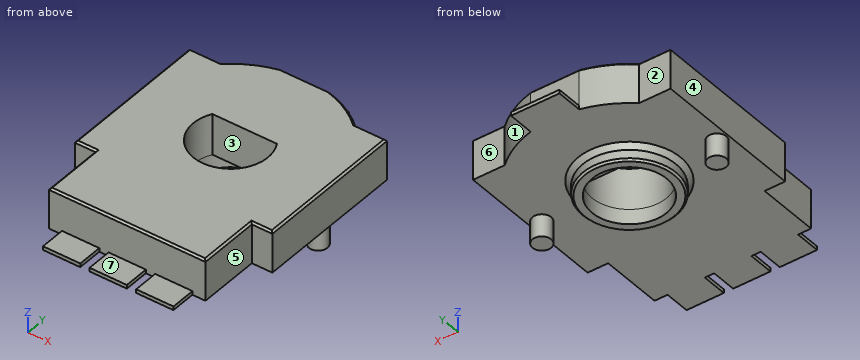
```python
from build123d import *

# Parameters (mm, degrees)
MODEL_R        = 0.5
MODEL_R_2      = 2.5
MODEL_R_3      = 2
EXTRUDE1_DEPTH = 2.2
SKETCH_W       = 1
SKETCH_H       = 1.35
EXTRUDE2_DEPTH = 0.2
SKETCH_2_R     = 2.5
SKETCH_2_R_2   = 2
EXTRUDE3_DEPTH = 0.8
SKETCH_3_R     = 0.5
EXTRUDE4_DEPTH = 1.2
CHAMFER1_SIZE  = 0.1
CHAMFER2_SIZE  = 0.25
CHAMFER3_SIZE  = 0.1
EXTRUDE5_START = -2.2
EXTRUDE5_DEPTH = 2.2


# Read off the part's stored shape, not the designer's step: Extrude5
with BuildPart() as part:
    # Model → Extrude1 (new body)
    # profile 1 of 5: a face of its own
    with BuildSketch(Plane.XY):
        with BuildLine():
            Line((0, 5.3), (-1.3, 5.3))
            ThreePointArc((-1.3, 5.3), (-2.523074038, 4.838811569), (-3.601388621, 4.1))
            Line((-3.601388621, 4.1), (-5.3, 4.1))
            Line((-5.3, 4.1), (-5.3, 0))
            Line((-5.3, 0), (-5.3, -4.05))
            Line((-5.3, -4.05), (-4.2, -4.05))
            Line((-4.2, -4.05), (-4.2, -7.35))
            Line((-4.2, -7.35), (0, -7.35))
            Line((0, -7.35), (4.2, -7.35))
            Line((4.2, -7.35), (4.2, -4.05))
            Line((4.2, -4.05), (5.3, -4.05))
            Line((5.3, -4.05), (5.3, 0))
            Line((5.3, 0), (5.3, 4.1))
            Line((5.3, 4.1), (3.601388621, 4.1))
            ThreePointArc((3.601388621, 4.1), (2.523074038, 4.838811569), (1.3, 5.3))
            Line((1.3, 5.3), (0, 5.3))
        make_face()
        with Locations((4.7, 0)):
            Circle(MODEL_R, mode=Mode.SUBTRACT)
        with Locations((-4.7, 0)):
            Circle(MODEL_R, mode=Mode.SUBTRACT)
        Circle(MODEL_R_2, mode=Mode.SUBTRACT)
    # profile 2 of 5: a face of its own
    with BuildSketch(Plane.XY):
        with Locations((-4.7, 0)):
            Circle(MODEL_R)
    # profile 3 of 5: a face of its own
    with BuildSketch(Plane.XY):
        with Locations((4.7, 0)):
            Circle(MODEL_R)
    # profile 4 of 5: a face of its own
    with BuildSketch(Plane.XY):
        Circle(MODEL_R_2)
        Circle(MODEL_R_3, mode=Mode.SUBTRACT)
    # profile 5 of 5: a face of its own
    with BuildSketch(Plane.XY):
        Circle(MODEL_R_3)
    extrude(amount=EXTRUDE1_DEPTH)

    # Sketch → Extrude2 (add)
    with BuildSketch(Plane.XY):
        Polygon((0, 6.7), (-1.3, 6.7), (-1.3, 5.3), (0, 5.3), (1.3, 5.3), (1.3, 6.7), align=None)
        with Locations((-2, -8.025)):
            Rectangle(SKETCH_W, SKETCH_H)
        with Locations((-3, -8.025)):
            Rectangle(SKETCH_W, SKETCH_H)
        Polygon((1, -8.7), (1, -7.35), (0, -7.35), (-1, -7.35), (-1, -8.7), (0, -8.7), align=None)
        with Locations((2, -8.025)):
            Rectangle(SKETCH_W, SKETCH_H)
        with Locations((3, -8.025)):
            Rectangle(SKETCH_W, SKETCH_H)
    extrude(amount=EXTRUDE2_DEPTH)

    # Sketch 2 → Extrude3 (add)
    with BuildSketch(Plane.XY):
        Circle(SKETCH_2_R)
        Circle(SKETCH_2_R_2, mode=Mode.SUBTRACT)
    extrude(amount=-EXTRUDE3_DEPTH)

    # Sketch 3 → Extrude4 (add)
    with BuildSketch(Plane.XY):
        with Locations((4.7, 0)):
            Circle(SKETCH_3_R)
        with Locations((-4.7, 0)):
            Circle(SKETCH_3_R)
    extrude(amount=-EXTRUDE4_DEPTH)

    # Chamfer1
    chamfer1_edges = [part.edges().sort_by_distance(p)[0] for p in [
        (-4.450694311, 4.1, 2.2),
        (-5.3, 0.025, 2.2),
        (-4.75, -4.05, 2.2),
        (-4.2, -5.7, 2.2),
        (0, -7.35, 2.2),
        (4.2, -5.7, 2.2),
        (0, 5.3, 2.2),
        (4.75, -4.05, 2.2),
        (5.3, 0.025, 2.2),
        (4.450694311, 4.1, 2.2),
        (2.523074038, 4.838811569, 2.2),
        (-2.523074038, 4.838811569, 2.2),
    ]]
    chamfer(chamfer1_edges, length=CHAMFER1_SIZE)

    # Chamfer2
    chamfer2_edges = [part.edges().sort_by_distance(p)[0] for p in [
        (-2.5, 0, 0),
    ]]
    chamfer(chamfer2_edges, length=CHAMFER2_SIZE)

    # Chamfer3
    chamfer3_edges = [part.edges().sort_by_distance(p)[0] for p in [
        (-2.5, 0, -0.8),
    ]]
    chamfer(chamfer3_edges, length=CHAMFER3_SIZE)

    # Extrude5 outline → Extrude5 (cut)
    with BuildSketch(Plane.XY.offset(2.2).offset(EXTRUDE5_START)):
        with BuildLine():
            ThreePointArc((-1.732050808, 1), (0, -2), (1.732050808, 1))
            Line((1.732050808, 1), (-1.732050808, 1))
        make_face()
    extrude(amount=EXTRUDE5_DEPTH, mode=Mode.SUBTRACT)


solid = part.part
```
CAD build for the part. Positions are in the model's coordinates, mm. Face numbers are marked on the shaded views. A direction names the side the tool comes from. Coordinates: 2 decimals unless noted, no trailing zeros. Write each loop counter-clockwise with the first axis right and the second up, starting at its lowest first coordinate (ties: lowest second). Pieces come first, ordered by that corner, then holes. Notation, with made-up numbers: (-4.5, -19) -> (35.5, -19) arc R22 ccw to (35.5, 8) -> close; hole circle Ø5 at (11.5, 45). An arc over 180 degrees is marked (long way). Return JSON: item names as keys, results as strings. Group by question number.
Q1. Cut at A-A, the plane z = 0.55. Give the cut face in (x, y), then the cut area to 3 significant figures.
Q2. Cut at B-B, the plane x = 0. Give the cut face in (y, z), then the cut area to 3 significant figures.
Q3. Cut at C-C, the plane y = -5. Give the cut face in (x, z), then the cut area to 3 significant figures.
Q4. Cut at D-D, the plane x = 4.7. Give the cut face in (y, z), then the cut area to 3 significant figures.
Q5. Drill centre lines: line 1 (Y direction, x = 1, z = -0.15); line 2 (X direction, y = 0, z = 1.2); line 3 (Z direction, x = -2.25, y = -4.5). Where is each one in solid material? Low to high.
Q6. Which spindle directions (+Z, -Z, +X, -X, +Y, -Y) get a long thin tool onto all of the face, cutting with end or side? Do the marked faces 5, 6 and 7. Say none if no direction does.
Q7. Pull direction X, two halves, no side cores. Call the marked faces 1, 2, 3 and 4: released by +X, released by -X, zero draft, split by the parting line, or undercut.
Q8. Flat gauge pins, fed straight in: pin 1 (1.5 mm diameter, centred on x = 0.5, y = 5.5, fed in from +Z); pin 2 (0.6 mm diameter, centred on x = -2, z = 1, fed in from -Y); pin 3 (2.5 mm diameter, centred on x = 0, y = 0, fed in from -Z); pin 4 (0.7 mm diameter, centred on x = 0, y = -8, fed in from +Z). Where does each tip first touch, or does it go through?
Returned:
{
 "1": {"outline": "(-5.3, -4.05) -> (-4.2, -4.05) -> (-4.2, -7.35) -> (4.2, -7.35) -> (4.2, -4.05) -> (5.3, -4.05) -> (5.3, 4.1) -> (3.6, 4.1) arc R5.46 ccw to (1.3, 5.3) -> (-1.3, 5.3) arc R5.46 ccw to (-3.6, 4.1) -> (-5.3, 4.1) -> close; hole (-1.73, 1) arc R2 ccw (long way) to (1.73, 1) -> close", "area": "110 mm2"},
 "2": {"outline": "(-8.7, 0) -> (-2.75, 0) -> (-2.5, -0.25) -> (-2.5, -0.7) -> (-2.4, -0.8) -> (-2, -0.8) -> (-2, 2.2) -> (-7.25, 2.2) -> (-7.35, 2.1) -> (-7.35, 0.2) -> (-8.7, 0.2) -> close; (1, 0) -> (2, 0) -> (2, -0.8) -> (2.4, -0.8) -> (2.5, -0.7) -> (2.5, -0.25) -> (2.75, 0) -> (6.7, 0) -> (6.7, 0.2) -> (5.3, 0.2) -> (5.3, 2.1) -> (5.2, 2.2) -> (1, 2.2) -> close", "area": "22.6 mm2"},
 "3": {"outline": "(-4.2, 0) -> (4.2, 0) -> (4.2, 2.1) -> (4.1, 2.2) -> (-4.1, 2.2) -> (-4.2, 2.1) -> close", "area": "18.5 mm2"},
 "4": {"outline": "(-4.05, 0) -> (-0.5, 0) -> (-0.5, -1.2) -> (0.5, -1.2) -> (0.5, 0) -> (4.1, 0) -> (4.1, 2.1) -> (4, 2.2) -> (-3.95, 2.2) -> (-4.05, 2.1) -> close", "area": "19.1 mm2"},
 "5": {"line 1": "y = -2.4 to -1.73, 1.73 to 2.4", "line 2": "x = -5.3 to -2, 2 to 5.3", "line 3": "z = 0 to 2.2"},
 "6": {"face 5": "+Z, -Z, +X, -Y", "face 6": "+Z, -Z, +X, +Y", "face 7": "+Z, +X, -X, -Y"},
 "7": {"face 1": "released by +X", "face 2": "zero draft", "face 3": "undercut", "face 4": "released by -X"},
 "8": {"pin 1": "stops at z = 2.2", "pin 2": "stops at y = -7.35", "pin 3": "stops at z = 0", "pin 4": "stops at z = 0.2"}
}
